```python
from build123d import *

# Parameters (mm, degrees)
F1_DEPTH = 6.35
F2_R     = 5.08
F5_D     = 5.08
F6_D     = 5.08
F7_R     = 1.26999


# Not quite as in the source:
# - a fillet or chamfer is up to 0.001 mm smaller than in the source, because OpenCascade refuses the exact size


with BuildPart() as f1:
    # F0 (on Front) → F1 (new body, symmetric)
    with BuildSketch(Plane.XZ):
        Polygon((-2.54, 0), (0, 0), (0, 18.3514992646), (-10.7314998529, 18.3514992646), (-10.7314998529, -20.8914992646), (-7.62, -20.8914992646), (-7.62, 15.176498382), (-2.54, 15.176498382), align=None)
    extrude(amount=F1_DEPTH, both=True)

    # F2
    f2_edges = [f1.edges().sort_by_distance(p)[0] for p in [
        (0, 0, 18.351499),
        (-10.7315, 0, 18.351499),
    ]]
    fillet(f2_edges, radius=F2_R)

    # F5 (through all)
    with Locations(Plane.XY.offset(18.3514992646)):
        with Locations((-5.3486400284, 0)):
            Hole(F5_D / 2)

    # F6 (through all)
    with Locations(Plane(origin=(-10.7314998529, 0, 0), x_dir=(0, -1, 0), z_dir=(-1, 0, 0))):
        with Locations((0, -9.9572697654)):
            Hole(F6_D / 2)

    # F7 (radius 1.27 in the source; OpenCascade refuses exactly that, so slightly less here)
    f7_edges = [f1.edges().sort_by_distance(p)[0] for p in [
        (0, 0, 0),
        (-2.54, 0, 0),
    ]]
    fillet(f7_edges, radius=F7_R)


solid = f1.part
```
Source: CAD feature listing. Evaluate the final solid. Frame: model axes, mm. A direction names the side the tool comes from. Round coordinates to 2 decimals unless told otherwise and drop trailing zeros. Loops run counter-clockwise (first coordinate to the right, second up) from the corner with the lowest first, then second, coordinate; pieces in that order, holes last. Notation, with made-up numbers: M 73.25,-28 L 97.25,-28 A12 cw 97.25,-10 Z; hole C 73,-25 d6. An arc over 180 degrees is marked long. Use a Markdown table: item, result. Add a question column.
1. Cut plane C-C, the plane x = -6.25. Output: boundary loops of the cut face in (y, z), and give its area (3 significant figures).
2. Contact query for flat-ended pins moving along their axis: pin 1 (1.5 mm diameter, centred on x = -5.5, y = -2.5, fed in from -Z); pin 2 (3 mm diameter, centred on y = 0, z = -16.5, fed in from +X); pin 3 (1 mm diameter, centred on x = -2, y = 0, fed in from +Z); pin 4 (3 mm diameter, centred on y = 0, z = -9.96, fed in from -X). Output: stop coordinate, or through.
3. Pull-direction query (X, two-part tool) for faces 3 (the flat face through (-7.62, -4, -3)), 4 (the cylindrical face through (-1.528, -0.089, 16.903)), 5 (the flat face through (-8, -6.35, 3)), 6 (the cylindrical face through (-7.867, -0.332, 10.094)); classes: +X half, -X half, draft (parallel to the pull), parting line (faces both ways), or undercut.
4. Ray query, line 1 along X through (y, z) = (0, 11); line 2 along X through (y, z) = (3.5, 13.5); line 3 along Z through (x, y) = (-5.75, 5). Return the intervals inside material, ascending. Write a range as [from, to].
5. Cut plane B-B, the plane y = -1.5. State how many separate pieces and enclosed holes the cut face has, and give its area (3 significant figures).
6. Cut plane A-A, the plane z = 3. Output: boundary loops of the cut face in (x, y), and give its area (3 significant figures).
7. Set-up query: faces 1 (the flat face through (-9, 0, -20.891)), 2 (the cylindrical face through (-2.178, 0.089, 0.382)). Return all of +Z, -Z, +X, -X, +Y, -Y with unobstructed straight access to the full face (end or side cutting, diameter ignored); none if empty.
Solution:
| question | item | result |
|---|---|---|
| 1 | outline | M -6.35,15.18 L -2.37,15.18 L -2.37,18.32 L -6.35,18.32 Z; M 2.37,15.18 L 6.35,15.18 L 6.35,18.32 L 2.37,18.32 Z |
| 1 | area | 25.0 mm2 |
| 2 | pin 1 | stops at z = 15.18 |
| 2 | pin 2 | stops at x = -7.62 |
| 2 | pin 3 | stops at z = 17.65 |
| 2 | pin 4 | passes through |
| 3 | face 3 | undercut |
| 3 | face 4 | +X half |
| 3 | face 5 | draft |
| 3 | face 6 | undercut |
| 4 | line 1 | x = [-10.73, -7.89], [-2.54, 0] |
| 4 | line 2 | x = [-10.73, -7.62], [-2.54, -0.01] |
| 4 | line 3 | z = [15.18, 18.35] |
| 5 | separate pieces | 3 |
| 5 | enclosed holes | 0 |
| 5 | area | 148 mm2 |
| 6 | outline | M -10.73,-6.35 L -7.62,-6.35 L -7.62,-1.14 A2.54 cw -7.62,1.14 L -7.62,6.35 L -10.73,6.35 Z; M -2.54,-6.35 L 0,-6.35 L 0,6.35 L -2.54,6.35 Z |
| 6 | area | 71.4 mm2 |
| 7 | face 1 | -Z, +X, -X, +Y, -Y |
| 7 | face 2 | -Z, +Y, -Y |
